Work out the finished part from the listing and answer in its coordinate system (mm). Face numbers are marked on the shaded views. A direction names the side the tool comes from. Coordinates: 2 decimals unless noted, no trailing zeros. Order: outer loops, then holes, each group sorted by start corner. A loop starts at its lowest first (then second) coordinate and runs counter-clockwise, first axis right, second up. Notation, with made-up numbers: (-34, 6) -> (6, 6) arc R22 ccw to (6, 17) -> close; hole circle Ø5 at (12.5, 41.25). An arc over 180 degrees is marked (long way). Write item = value, one per line. Start each with the question number.
Q1. The part is cut by section D-D, the plane x = 13. Determine the outline of the cut face in (y, z) (3 decimals), plus the area to 3 significant figures.
Q2. The part is cut by section B-B, the plane z = 5. Determine the outline of the cut face in (x, y), plus the area to 3 significant figures.
Q3. Flat-ended cylindrical pins translate along their axes: pin 1 (3 mm diameter, centred on y = -8.5, z = 7.5, fed in from -X); pin 2 (1 mm diameter, centred on y = -11.5, z = 7, fed in from -X); pin 3 (4 mm diameter, centred on y = -6.5, z = 1.5, fed in from +X). Find the tip coordinate at first contact, or state that the pin passes through.
Q4. For a pull along Y with two mould halves and no side action, classify the marked faces 5, 6, 7 and 8 as +Y half, -Y half, draft (parallel to the pull), parting line (faces both ways), or undercut.
Q5. The part is cut by section A-A, the plane x = 0. Determine the outline of the cut face in (y, z) (3 decimals), plus the area to 3 significant figures.
Q6. Which of the six approach directions +Z, -Z, +X, -X, +Y, -Y give full straight-line access (tool end or side, diameter ignored) to the marked faces 1, 2, 3 and 4?
Q7. The part is cut by section C-C, the plane y = -9.5. Determine the outline of the cut face in (x, z) (3 decimals).
Q8. Straight lines are drawn through the part: L1, parallel to Y at x = 0, z = 6; L2, parallel to Y at x = 0, z = 2.5 (3 decimals); L3, parallel to Z at x = 12, y = 5. For each, find the intervals that lie inside material, in ascending order. Write a range as from..to.
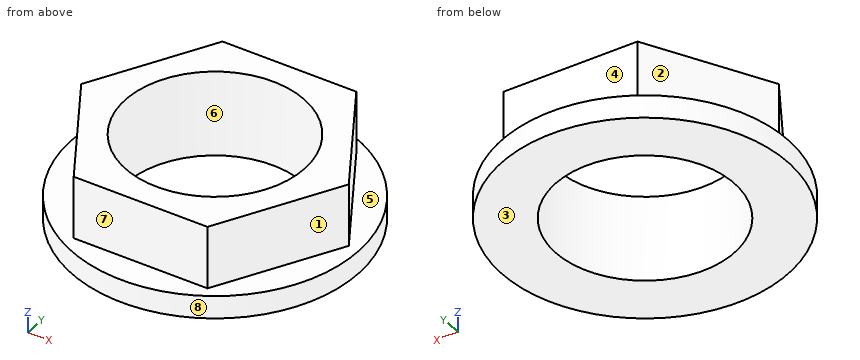
```python
from build123d import *

# Parameters (mm, degrees)
F0_R     = 9.906
F1_DEPTH = 9.525
F2_R     = 15.875
F2_R_2   = 9.906
F3_DEPTH = 2.54


with BuildPart() as f1:
    # F0 (on Top) → F1 (new body)
    with BuildSketch(Plane.XY):
        Polygon((7.332348, 12.7), (-7.332348, 12.7), (-14.664697, 0), (-7.332348, -12.7), (7.332348, -12.7), (14.664697, 0), align=None)
        Circle(F0_R, mode=Mode.SUBTRACT)
    extrude(amount=F1_DEPTH)

    # F2 (on Top) → F3 (join)
    with BuildSketch(Plane.XY):
        Circle(F2_R)
        Circle(F2_R_2, mode=Mode.SUBTRACT)
    extrude(amount=F3_DEPTH)


solid = f1.part
```
Model answer:
q1.outline = (-9.111, 0) -> (9.111, 0) -> (9.111, 2.54) -> (2.883, 2.54) -> (2.883, 9.525) -> (-2.883, 9.525) -> (-2.883, 2.54) -> (-9.111, 2.54) -> close
q1.area = 86.6 mm2
q2.outline = (-14.66, 0) -> (-7.33, -12.7) -> (7.33, -12.7) -> (14.66, 0) -> (7.33, 12.7) -> (-7.33, 12.7) -> close; hole circle Ø19.81 at (0, 0)
q2.area = 250 mm2
q3.pin_1 = -10.62
q3.pin_2 = -8.31
q3.pin_3 = 15.22
q4.face_5 = draft
q4.face_6 = undercut
q4.face_7 = -Y half
q4.face_8 = parting line
q5.outline = (-15.875, 0) -> (-9.906, 0) -> (-9.906, 9.525) -> (-12.7, 9.525) -> (-12.7, 2.54) -> (-15.875, 2.54) -> close; (9.906, 0) -> (15.875, 0) -> (15.875, 2.54) -> (12.7, 2.54) -> (12.7, 9.525) -> (9.906, 9.525) -> close
q5.area = 69.4 mm2
q6.face_1 = +Z, +X, -Y
q6.face_2 = +Z, -X, +Y
q6.face_3 = -Z, +X, -X, +Y, -Y
q6.face_4 = +Z, +X, -X, +Y
q7.outline = (-12.719, 0) -> (-2.807, 0) -> (-2.807, 9.525) -> (-9.18, 9.525) -> (-9.18, 2.54) -> (-12.719, 2.54) -> close; (2.807, 0) -> (12.719, 0) -> (12.719, 2.54) -> (9.18, 2.54) -> (9.18, 9.525) -> (2.807, 9.525) -> close
q8.L1 = -12.7..-9.91, 9.91..12.7
q8.L2 = -15.875..-9.906, 9.906..15.875
q8.L3 = 0..2.54
